Verification items for the finished model (mm, model axes). A direction names the side the tool comes from. Round coordinates to 2 decimals unless told otherwise and drop trailing zeros. Order: outer loops, then holes, each group sorted by start corner. A loop starts at its lowest first (then second) coordinate and runs counter-clockwise, first axis right, second up. Notation, with made-up numbers: (15, -7) -> (68, -7) arc R21 cw to (68, 31) -> close; hole circle Ø7 at (-34.75, 57.25). An arc over 180 degrees is marked (long way). Put each result on its own line as item: value.
from build123d import *

# Parameters (mm, degrees)
SKETCH_1_R      = 1.5
EXTRUDE_1_DEPTH = 2.4
SKETCH_4_R      = 2.4
SKETCH_4_R_2    = 1.5
EXTRUDE_3_DEPTH = 1.2
FILLET_5_R      = 0.3


with BuildPart() as part:
    # 草图1 → 凸台-拉伸1 (new body)
    with BuildSketch(Plane(origin=(0, 0, 0), x_dir=(1, 0, 0), z_dir=(0, 1, 0))):
        Polygon((0, 3.175426481), (-2.75, 1.58771324), (-2.75, -1.58771324), (0, -3.175426481), (2.75, -1.58771324), (2.75, 1.58771324), align=None)
        with Locations(Location((0, 0, 0), (0, 0, 270))):
            Circle(SKETCH_1_R, mode=Mode.SUBTRACT)
    extrude(amount=EXTRUDE_1_DEPTH)

    # 草图3 → 切除-旋转7 (revolve, cut)
    with BuildSketch(Plane(origin=(0, 0, 0), x_dir=(0, 0, -1), z_dir=(1, 0, 0))):
        Polygon((0.384303775, 7.2), (4.083483307, 7.2), (4.083483307, -4.8), (0.297701235, -4.8), (0.297701235, -4.284366336), (3.464101615, 1.2), (0.384303775, 6.534366336), align=None)
    revolve(axis=Axis((0, 2.4, 0), (0, -1, 0)), mode=Mode.SUBTRACT)

    # 草图4 → 凸台-拉伸3 (add)
    with BuildSketch(Plane(origin=(0, 2.4, 0), x_dir=(1, 0, 0), z_dir=(0, 1, 0))):
        with Locations(Location((0, 0, 0), (0, 0, 270))):
            Circle(SKETCH_4_R)
        with Locations(Location((0, 0, 0), (0, 0, 270))):
            Circle(SKETCH_4_R_2, mode=Mode.SUBTRACT)
    extrude(amount=EXTRUDE_3_DEPTH)

    # 圆角5
    fillet_5_edges = [part.edges().sort_by_distance(p)[0] for p in [
        (0, 3.6, -2.4),
    ]]
    fillet(fillet_5_edges, radius=FILLET_5_R)


solid = part.part
Item 1: Section check C-C on y = 2.3. Record the boundary of the cut face in (x, z).
Check sheet entries:
outline: (-2.75, -0.66) arc R2.83 ccw to (-1.95, -2.05) -> (-0.8, -2.71) arc R2.83 ccw to (0.8, -2.71) -> (1.95, -2.05) arc R2.83 ccw to (2.75, -0.66) -> (2.75, 0.66) arc R2.83 ccw to (1.95, 2.05) -> (0.8, 2.71) arc R2.83 ccw to (-0.8, 2.71) -> (-1.95, 2.05) arc R2.83 ccw to (-2.75, 0.66) -> close; hole circle Ø3 at (0, 0)
Item 2: Release check for a two-part mould opening along Z. For faces 1 (the cylindrical face through (0.45, 1.77, 1.43)), 2 (the flat face through (-1.4, 3.6, 0.9)), 3 (the conical face through (2.49, 0.2, -1.46)) record: +Z half, -Z half, draft (parallel to the pull), parting line (faces both ways), or undercut.
Check sheet entries:
face 1: undercut
face 2: draft
face 3: -Z half
Item 3: Section check B-B on y = 1.55. Record the boundary of the cut face in (x, z).
Check sheet entries:
outline: (-2.75, -1.59) -> (0, -3.18) -> (2.75, -1.59) -> (2.75, 1.59) -> (0, 3.18) -> (-2.75, 1.59) -> close; hole circle Ø3 at (0, 0)
Item 4: Section check A-A on z = 0. Record the boundary of the cut face in (x, y), then the cut area to 3 significant figures.
Check sheet entries:
outline: (-2.75, 0) -> (-1.5, 0) -> (-1.5, 3.6) -> (-2.1, 3.6) arc R0.3 ccw to (-2.4, 3.3) -> (-2.4, 2.4) -> (-2.75, 2.4) -> close; (1.5, 0) -> (2.75, 0) -> (2.75, 2.4) -> (2.4, 2.4) -> (2.4, 3.3) arc R0.3 ccw to (2.1, 3.6) -> (1.5, 3.6) -> close
area: 8.12 mm^2
Item 5: Gauge pin test, flat ends, axial feed: pin 1 Ø1.5 at (x, y) = (1.5, 1.5) entering from +Z; pin 2 Ø1.8 at (x, z) = (0, 0) entering from -Y. Record the tip position at first contact, or that the pin passes through.
Check sheet entries:
pin 1: stops at z = 2.74
pin 2: passes through
Item 6: Tool access check on faces 4 (the cylindrical face through (2.024, 2.844, 1.29)), 5 (the conical face through (-2.49, 2.21, 1.45)). Record the directions out of +Z, -Z, +X, -X, +Y, -Y that give a thin tool (end or side, any length) a straight path to the whole face; none if there is none.
Check sheet entries:
face 4: +Y
face 5: +Z, -X, +Y
Item 7: Material ranges on L1, parallel to X at y = 2.85, z = 0; L2, parallel to X at y = 2.35, z = 0, recorded low to high. Write a range as [from, to].
Check sheet entries:
L1: x = [-2.4, -1.5], [1.5, 2.4]
L2: x = [-2.75, -1.5], [1.5, 2.75]
